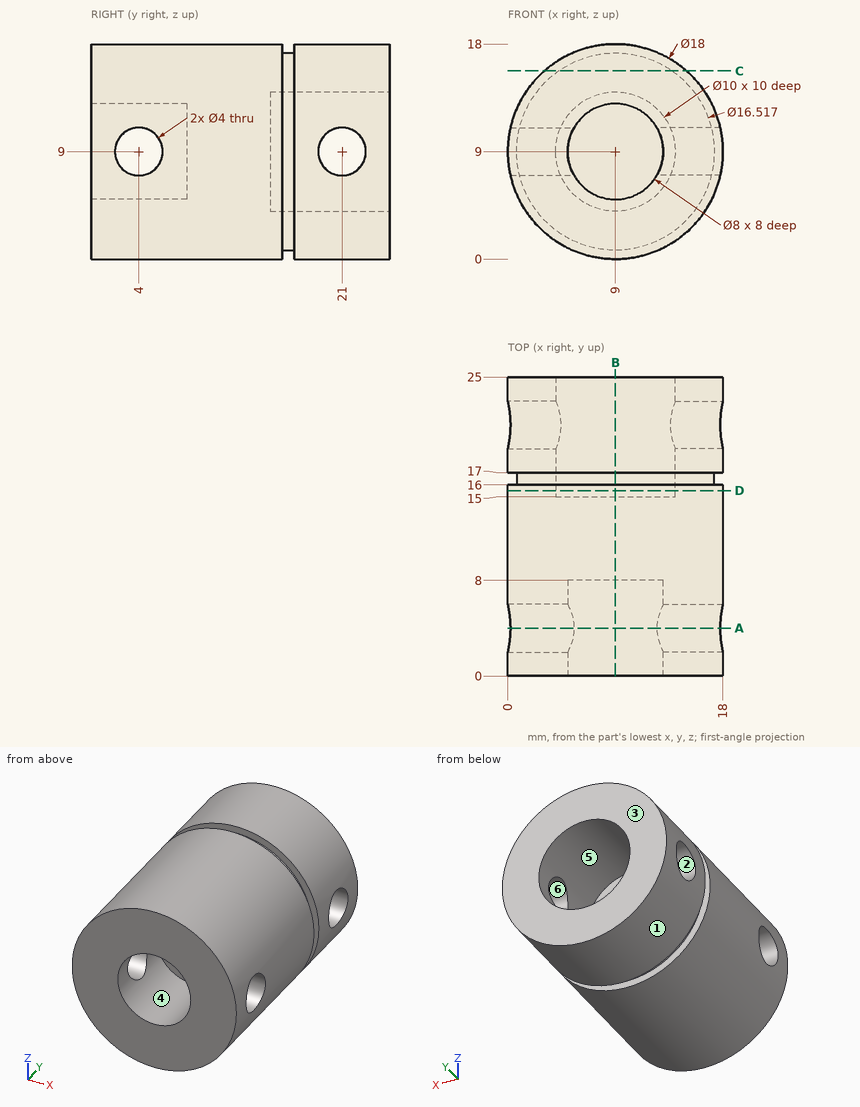
Check sheet for the drawn part. Datum: minimum x, y, z corner. Units: mm. A direction names the side the tool comes from. Coordinates: 2 decimals unless noted, no trailing zeros. Order: outer loops, then holes, each group sorted by start corner. A loop starts at its lowest first (then second) coordinate and runs counter-clockwise, first axis right, second up. Notation, with made-up numbers: M 52,-16 L 97,-16 A34 cw 97,22 Z; hole C 0.25,57.25 d9. An arc over 180 degrees is marked long. One line per item, written item: value. Start each with the question number.
Item 1: Mould release check, pull along Z, two halves, no side actions. Record for the marked faces 1, 2 and 3: released by +Z, released by -Z, zero draft, split by the parting line, or undercut.
Item 2: Sectioned sample at D-D (y = 15.5). Enter the section's corners in (x, z), then the cut area to 3 significant figures.
Item 3: Sectioned sample at B-B (x = 9). Enter the section's corners in (y, z).
Item 4: Scan lines: probe 1 along Z at (x, y) = (9, 24.25); probe 2 along X at (y, z) = (15.5, 9.25); probe 3 along Y at (x, z) = (2, 8.75). Record each from-to range of solid material in increasing order.
Item 5: Sectioned sample at A-A (y = 4). Enter the section's corners in (x, z) (1 decimal), then the cut area to 3 significant figures.
Item 6: Sectioned sample at C-C (z = 15.75). Enter the section's corners in (x, y), then the cut area to 3 significant figures.
Item 7: Access from +Z, -Z, +X, -X, +Y, -Y to the whole of each face (thin tool, end or side, straight path). Record for the marked faces 4, 5 and 6.
Item 8: Gauge pin test, flat ends, axial feed: pin 1 (3 mm diameter, centred on y = 16.5, z = 5.5, fed in from +X) (3 decimals); pin 2 (10 mm diameter, centred on y = 20.5, z = 15.5, fed in from +X); pin 3 (4 mm diameter, centred on x = 12.5, y = 14.5, fed in from +Z). Record the tip position at first contact, or that the pin passes through.
Conclusion:
1. face 1: split by the parting line
1. face 2: undercut
1. face 3: zero draft
2. outline: C 9,9 d18; hole C 9,9 d10
2. area: 176 mm^2
3. outline: M 0,0 L 16,0 L 16,0.74 L 17,0.74 L 17,0 L 25,0 L 25,4 L 15,4 L 15,14 L 25,14 L 25,18 L 17,18 L 17,17.26 L 16,17.26 L 16,18 L 0,18 L 0,13 L 8,13 L 8,5 L 0,5 Z
4. probe 1: z = 0 to 4, 14 to 18
4. probe 2: x = 0 to 4.01, 13.99 to 18
4. probe 3: y = 0 to 2.02, 5.98 to 19.02, 22.98 to 25
5. outline: M 0.2,7 A9 ccw 17.8,7 L 12.5,7 A4 cw 5.5,7 Z; M 0.2,11 L 5.5,11 A4 cw 12.5,11 L 17.8,11 A9 ccw Z
5. area: 163 mm^2
6. outline: M 3.05,0 L 14.95,0 L 14.95,16 L 13.76,16 L 13.76,17 L 14.95,17 L 14.95,25 L 3.05,25 L 3.05,17 L 4.24,17 L 4.24,16 L 3.05,16 Z
6. area: 295 mm^2
7. face 4: -Y
7. face 5: +Y
7. face 6: +X, -X
8. pin 1: stops at x = 17.755
8. pin 2: stops at x = 17.86
8. pin 3: stops at z = 17.87
